The drawing under review shows one solid part. Ordinate dimensions are in mm from its lowest x, y, z. Coordinates: 2 decimals unless noted, no trailing zeros. Loops run counter-clockwise (first coordinate to the right, second up) from the corner with the lowest first, then second, coordinate; pieces in that order, holes last. Notation, with made-up numbers: (60, -24.75) - (79, -24.75) arc R22 cw to (79, -14.75) - close; hole circle Ø5 at (41, -34). An arc over 180 degrees is marked (long way). Answer as a JSON object with one key per item and string values. Group by question number.
Item 1: Mouldability with a two-part tool opening along Y and no side actions: class the marked faces 1, 2 and 3 as released by +Y, released by -Y, zero draft, split by the parting line, or undercut.
Item 2: We need section A-A (z = 24). Give the boundary of the cut face in (x, y) (1 decimal).
Item 3: To check wall thickness, follow line 1 (X direction, y = 14, z = 12); line 2 (X direction, y = 22.5, z = 61.5) (1 decimal); line 3 (Z direction, x = 24, y = 12) (1 decimal). State the ranges of each line that lie inside material, in increasing order.
Item 4: Clearance check with flat-ended pins moving along their axes: pin 1 (3 mm diameter, centred on y = 20, z = 22, fed in from +X); pin 2 (6 mm diameter, centred on y = 21.5, z = 35, fed in from -X) (1 decimal); pin 3 (6 mm diameter, centred on y = 22.5, z = 40.5, fed in from +X). State where each tip first meets the part, or that it passes through.
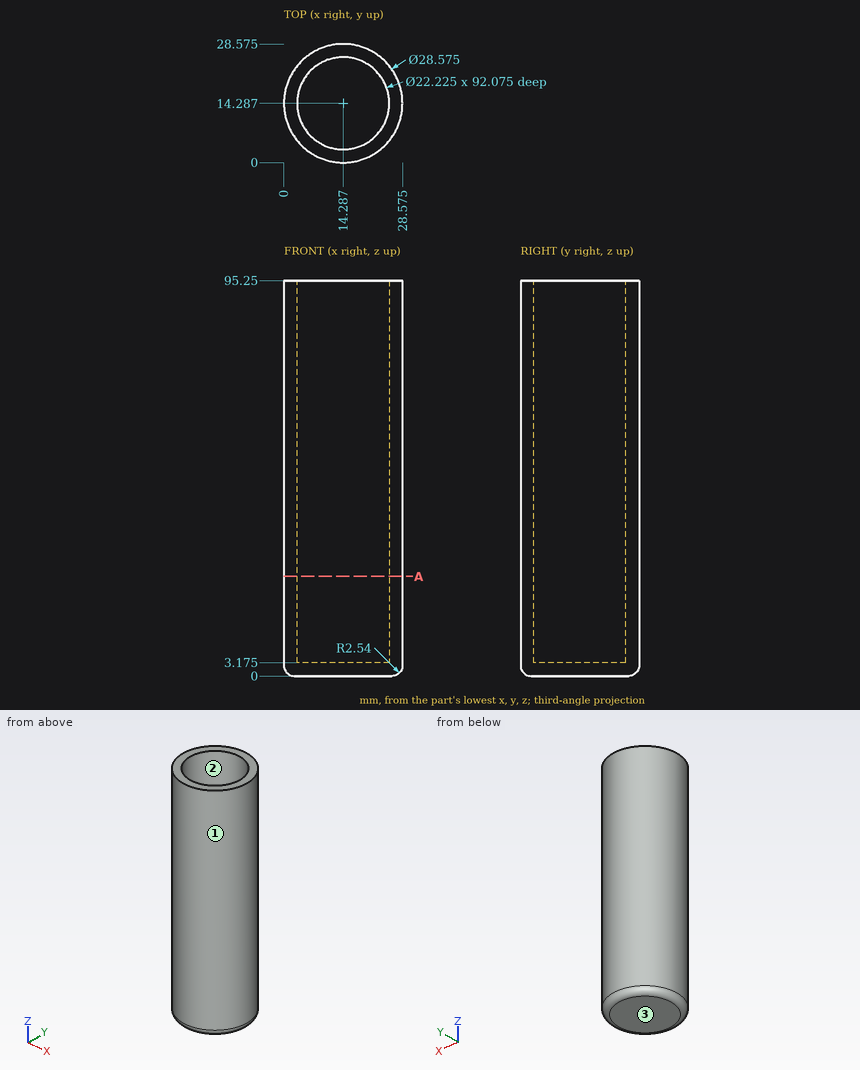
Check sheet entries:
{
 "1": {"face 1": "split by the parting line", "face 2": "undercut", "face 3": "zero draft"},
 "2": {"outline": "circle Ø28.6 at (14.3, 14.3); hole circle Ø22.2 at (14.3, 14.3)"},
 "3": {"line 1": "x = 0 to 3.18, 25.4 to 28.57", "line 2": "x = 2.6 to 6.8, 21.8 to 26", "line 3": "z = 0 to 3.2"},
 "4": {"pin 1": "stops at x = 27.94", "pin 2": "stops at x = 0.6", "pin 3": "stops at x = 27.59"}
}
